from build123d import *

# Parameters (mm, degrees)
EXTRUDE_1_DEPTH      = 25
EXTRUDE_1_DEPTH_BACK = 25
SKETCH_2_W           = 30
SKETCH_2_H           = 3
EXTRUDE_2_DEPTH      = 10
SKETCH_3_R           = 1.65
CUT_EXTRUDE_1_DEPTH  = 3


with BuildPart() as part:
    # 草图1 → 凸台-拉伸1 (new, two sides: drawn at the far end of the back side and taken through both)
    with BuildSketch(Plane.XY.offset(-EXTRUDE_1_DEPTH_BACK)):
        Polygon((-10, 55), (-15, 55), (-15, 0), (15, 0), (15, 21.823879459), (12.267155857, 25.450486128), (7.475342796, 21.839595989), (-11.782737945, 47.395932311), (-6.990924884, 51.00682245), align=None)
    extrude(amount=EXTRUDE_1_DEPTH + EXTRUDE_1_DEPTH_BACK)

    # 草图2 → 凸台-拉伸2 (add)
    with BuildSketch(Plane.XY.offset(25)):
        with Locations((0, 1.5)):
            Rectangle(SKETCH_2_W, SKETCH_2_H)
    extrude_2 = extrude(amount=EXTRUDE_2_DEPTH)

    # 草图3 → 切除-拉伸1 (cut)
    with BuildSketch(Plane(origin=(0, 3, 0), x_dir=(1, 0, 0), z_dir=(0, 1, 0))):
        with Locations(Location((0, -30, 0), (0, 0, 270))):
            Circle(SKETCH_3_R)
    cut_extrude_1 = extrude(amount=-CUT_EXTRUDE_1_DEPTH, mode=Mode.SUBTRACT)

    # 镜向1: 凸台-拉伸2, 切除-拉伸1 across plane
    add(extrude_2.mirror(Plane.XY))
    add(cut_extrude_1.mirror(Plane.XY), mode=Mode.SUBTRACT)


solid = part.part
Source: CAD feature listing. Evaluate the final solid. Frame: model axes, mm. A direction names the side the tool comes from. Give positions to 0.01 mm unless a question says otherwise; leave off trailing zeros. Write each loop counter-clockwise with the first axis right and the second up, starting at its lowest first coordinate (ties: lowest second). Pieces come first, ordered by that corner, then holes. Notation, with made-up numbers: M 68.25,-20 L 122.25,-20 A16 ccw 122.25,7 Z; hole C 89.25,4 d9. An arc over 180 degrees is marked long. Return JSON: item names as keys, results as strings. Group by question number.
1) Set-up query: faces 1 (the face through (-9.42, 49.176, -0.35)), 2 (the face through (-8.474, 52.975, -0.35)), 3 (the face through (-4, 24, -25)), 4 (the face through (-4, 24, 25)), 5 (the face through (9.905, 23.67, -0.35)). Return all of +Z, -Z, +X, -X, +Y, -Y with unobstructed straight access to the full face (end or side cutting, diameter ignored); none if empty.
2) Pull-direction query (Z, two-part tool) for faces 6 (the face through (0, 3, -28)), 7 (the face through (0, 2, 35)), 8 (the face through (0.07, 1.52, -28.35)); classes: pulls with the +Z half, pulls with the -Z half, needs draft (parallel to the pull), parting line crosses it, or undercut.
3) Cut plane B-B, the plane y = 24. Output: boundary loops of the cut face in (x, z).
4) Cut plane D-D, the plane z = -14.5. Output: boundary loops of the cut face in (x, y), plus the area to 3 significant figures.
5) Cut plane C-C, the plane x = 0. Output: boundary loops of the cut face in (y, z).
6) Material intervals for line 1 along X through (y, z) = (1.65, -30); line 2 along Z through (x, y) = (3.5, 15); line 3 along Y through (x, z) = (-9.75, 4.5), sorted ascending. Write a range as [from, to].
7) Pin query (flat end, axial travel): P1, Ø12, axis at x = -3, y = 7.5, coming from the +Z side; P2, Ø4.5, axis at x = 0, z = -30, coming from the +Y side; P3, Ø8, axis at x = 4.5, y = 22.5, coming from the -Z side; P4, Ø11, axis at x = 6.5, z = -29, coming from the +Y side. Return the tip coordinate at first contact, or that it passes through.
8) Cut plane A-A, the plane z = 30. Output: boundary loops of the cut face in (x, y).
Recorded:
{
 "1": {"face 1": "+Z, -Z, +X", "face 2": "+Z, -Z, +X, +Y", "face 3": "-Z, +X, -X, +Y", "face 4": "+Z, +X, -X, +Y", "face 5": "+Z, -Z, +Y"},
 "2": {"face 6": "needs draft", "face 7": "pulls with the +Z half", "face 8": "undercut"},
 "3": {"outline": "M -15,-25 L 5.85,-25 L 5.85,25 L -15,25 Z; M 10.34,-25 L 13.36,-25 L 13.36,25 L 10.34,25 Z"},
 "4": {"outline": "M -15,0 L 15,0 L 15,21.82 L 12.27,25.45 L 7.48,21.84 L -11.78,47.4 L -6.99,51.01 L -10,55 L -15,55 Z", "area": "1,040 mm²"},
 "5": {"outline": "M 0,-35 L 3,-35 L 3,-31.65 L 0,-31.65 Z; M 0,-28.35 L 3,-28.35 L 3,-25 L 31.76,-25 L 31.76,25 L 3,25 L 3,28.35 L 0,28.35 Z; M 0,31.65 L 3,31.65 L 3,35 L 0,35 Z"},
 "6": {"line 1": "x = [-15, -1.65], [1.65, 15]", "line 2": "z = [-25, 25]", "line 3": "y = [0, 44.7], [48.93, 54.67]"},
 "7": {"P1": "stops at z = 35", "P2": "stops at y = 3", "P3": "stops at z = -25", "P4": "stops at y = 28.14"},
 "8": {"outline": "M -15,0 L -1.65,0 L -1.65,3 L -15,3 Z; M 1.65,0 L 15,0 L 15,3 L 1.65,3 Z"}
}
